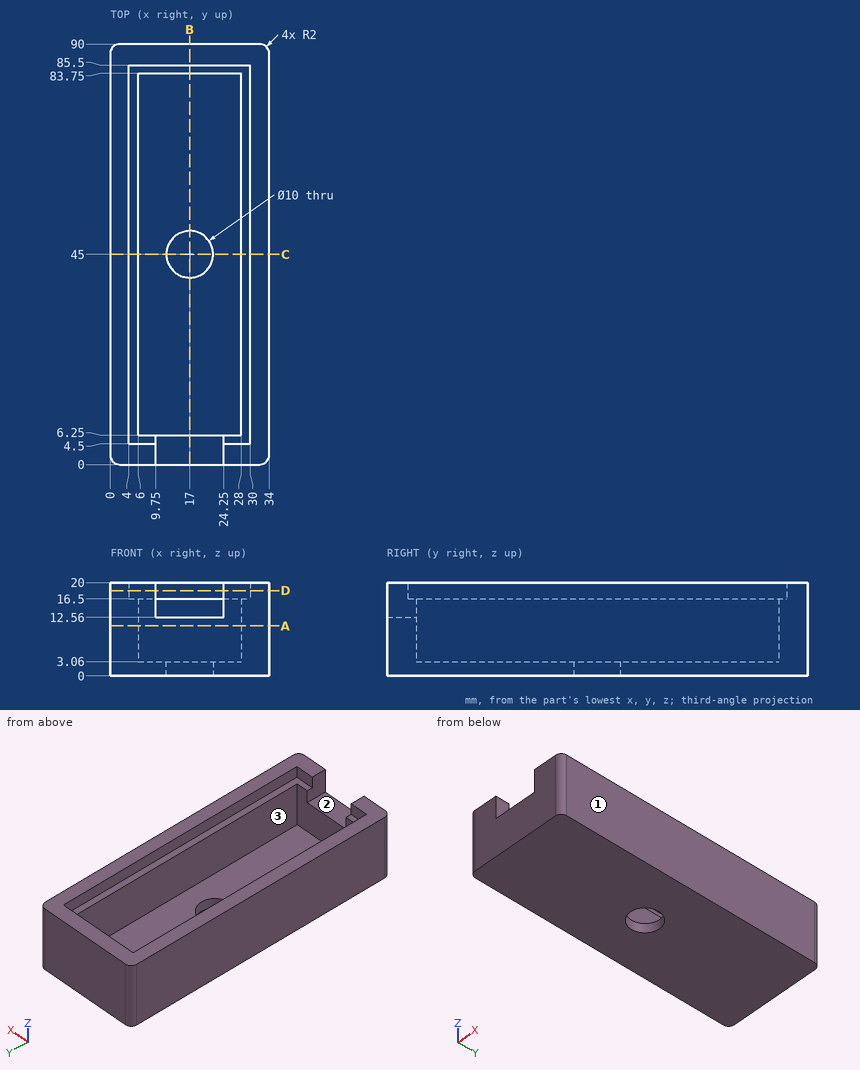
Design review of the part shown in the three views and the two pictorial views. Dimensions are in mm from the part's minimum x, y and z. A direction names the side the tool comes from. Round coordinates to 2 decimals unless told otherwise and drop trailing zeros. Loops run counter-clockwise (first coordinate to the right, second up) from the corner with the lowest first, then second, coordinate; pieces in that order, holes last. Notation, with made-up numbers: (-21.75, 10.5) -> (10.25, 10.5) arc R35 cw to (10.25, 44.5) -> close; hole circle Ø3 at (-3.75, 42). An arc over 180 degrees is marked (long way). Answer as a JSON object with one key per item and string values. Group by question number.
1) We need section C-C on y = 45. Write out the cut boundary in (x, z), then the cut area to 3 significant figures.
2) For line 1 (Y direction, x = 27, z = 9.5); line 2 (Y direction, x = 17, z = 1.75); line 3 (X direction, y = 20, z = 6.75), list the stretches that pass through material, from the lowest coordinate up. Write a range as [from, to].
3) We need section A-A on z = 10.75. Write out the cut boundary in (x, y).
4) We need section B-B on x = 17. Write out the cut boundary in (y, z), then the cut area to 3 significant figures.
5) For pin 1 Ø2 at (x, z) = (15, 13.5) entering from -Y; pin 2 Ø3 at (x, y) = (16.5, 3) entering from +Z; pin 3 Ø1.5 at (x, y) = (16, 19) entering from +Z; pin 4 Ø12 at (x, y) = (23.5, 48.5) entering from +Z, all flat-tipped, find the tip position at first contact; note any pin that passes through.
6) For the marked faces 1, 2 and 3, list the 3-axis set-ups (+Z, -Z, +X, -X, +Y, -Y) from which the entire face can be reached by the end or side of a thin tool; tool diameter is ignored.
7) We need section D-D on z = 18.25. Write out the cut boundary in (x, y), then the cut area to 3 significant figures.
Result set:
{
 "1": {"outline": "(0, 0) -> (12, 0) -> (12, 3.06) -> (6, 3.06) -> (6, 16.5) -> (4, 16.5) -> (4, 20) -> (0, 20) -> close; (22, 0) -> (34, 0) -> (34, 20) -> (30, 20) -> (30, 16.5) -> (28, 16.5) -> (28, 3.06) -> (22, 3.06) -> close", "area": "263 mm²"},
 "2": {"line 1": "[0, 6.25], [83.75, 90]", "line 2": "[0, 40], [50, 90]", "line 3": "[0, 6], [28, 34]"},
 "3": {"outline": "(0, 2) arc R2 ccw to (2, 0) -> (32, 0) arc R2 ccw to (34, 2) -> (34, 88) arc R2 ccw to (32, 90) -> (2, 90) arc R2 ccw to (0, 88) -> close; hole (6, 6.25) -> (28, 6.25) -> (28, 83.75) -> (6, 83.75) -> close"},
 "4": {"outline": "(0, 0) -> (40, 0) -> (40, 3.06) -> (6.25, 3.06) -> (6.25, 12.56) -> (0, 12.56) -> close; (50, 0) -> (90, 0) -> (90, 20) -> (85.5, 20) -> (85.5, 16.5) -> (83.75, 16.5) -> (83.75, 3.06) -> (50, 3.06) -> close", "area": "404 mm²"},
 "5": {"pin 1": "y = 0", "pin 2": "z = 12.56", "pin 3": "z = 3.06", "pin 4": "z = 16.5"},
 "6": {"face 1": "+Z, -Z, +X, +Y, -Y", "face 2": "+Z, -Y", "face 3": "+Z"},
 "7": {"outline": "(0, 2) arc R2 ccw to (2, 0) -> (9.75, 0) -> (9.75, 4.5) -> (4, 4.5) -> (4, 85.5) -> (30, 85.5) -> (30, 4.5) -> (24.25, 4.5) -> (24.25, 0) -> (32, 0) arc R2 ccw to (34, 2) -> (34, 88) arc R2 ccw to (32, 90) -> (2, 90) arc R2 ccw to (0, 88) -> close", "area": "885 mm²"}
}
